Here's how the part is built. I have some questions about the finished solid (model axes, mm). A direction names the side the tool comes from. Coordinates: 2 decimals unless noted, no trailing zeros. Write each loop counter-clockwise with the first axis right and the second up, starting at its lowest first coordinate (ties: lowest second). Pieces come first, ordered by that corner, then holes. Notation, with made-up numbers: M -18,-26 L 26,-26 A30 cw 26,11 Z; hole C -29.75,-35.75 d7. An arc over 180 degrees is marked long. Use one line per item in the form item = value. Start each with the question number.
1. I want a section at A-A, the plane z = 0. List the corners of the cut face in (x, y) for me.
2. I want a section at B-B, the plane y = 3.1. List the corners of the cut face in (x, z) for me, plus the area to 3 significant figures.
3. On a 3-axis mill with a long thin cutter (end or side, diameter ignored), from which of +Z, -Z, +X, -X, +Y, -Y can I reach the whole of each face in a straight line? I mean faces 4 (the face through (-164.45, 1.29, -2.54)), 5 (the face through (-61.05, 2.48, -0.25)). Say none if no direction works.
4. Thinking about a two-plate mould opening in Z: for faces 1 (the face through (-170.5, 2.105, 0.1)), 2 (the face through (-115, 0.505, 0)), 3 (the face through (-116, 2, -6)), which applies, released by +Z, released by -Z, zero draft, split by the parting line, or undercut?
5. I'm going to push flat-ended pins straight in: pin 1 Ø4.5 at (x, z) = (-62.95, 0) entering from -Y; pin 2 Ø2.5 at (x, z) = (-168.43, 0) entering from -Y; pin 3 Ø5.5 at (x, z) = (-168.43, 0) entering from -Y. Where does each tip first touch, or does it pass through?
6. Please list where these lines run through material, in increasing order: line 1 along X through (y, z) = (1.65, 0); line 2 along X through (y, z) = (2.8, 0.25); line 3 along Z through (x, y) = (-169, 4.15). Write a range as [from, to].
from build123d import *

# Parameters (mm, degrees)
SKETCH1_R           = 2.4
BOSS_EXTRUDE1_DEPTH = 5
SKETCH2_R           = 5.9
CUT_EXTRUDE1_DEPTH  = 2
SCALE1_SCALE        = 0.8


with BuildPart() as part:
    # Sketch1 → Boss-Extrude1 (new body)
    with BuildSketch(Plane(origin=(0, 0, 0), x_dir=(1, 0, 0), z_dir=(0, 1, 0))):
        with BuildLine():
            Line((-181.84579044, 7.5), (-50, 7.5))
            ThreePointArc((-50, 7.5), (-42.5, 0), (-50, -7.5))
            Line((-50, -7.5), (-181.84579044, -7.5))
            ThreePointArc((-181.84579044, -7.5), (-189.34579044, 0), (-181.84579044, 7.5))
        make_face()
        with Locations(Location((-181.84579044, 0, 0), (0, 0, 270))):
            Circle(SKETCH1_R, mode=Mode.SUBTRACT)
        with Locations(Location((-50, 0, 0), (0, 0, 270))):
            Circle(SKETCH1_R, mode=Mode.SUBTRACT)
    extrude(amount=BOSS_EXTRUDE1_DEPTH)

    # Sketch2 → Cut-Extrude1 (cut)
    with BuildSketch(Plane.XZ):
        with Locations(Location((-181.84579044, 0, 0), (0, 0, 270))):
            Circle(SKETCH2_R)
    extrude(amount=-CUT_EXTRUDE1_DEPTH, mode=Mode.SUBTRACT)


with BuildPart() as part_1:
    # Scale1: scaled about (-114.766854611, 2.52630438, 0)
    add(part.part.scale(SCALE1_SCALE).moved(Location((-22.953370922, 0.505260876, 0))))


solid = part_1.part
Answer list:
q1.outline = M -174.43,0.51 L -173.15,0.51 L -173.15,2.11 L -170.35,2.11 L -170.35,4.51 L -174.43,4.51 Z; M -166.51,2.11 L -163.71,2.11 L -163.71,0.51 L -64.87,0.51 L -64.87,4.51 L -166.51,4.51 Z; M -61.03,0.51 L -56.95,0.51 L -56.95,4.51 L -61.03,4.51 Z
q2.outline = M -168.43,-6 L -62.95,-6 A6 ccw -62.95,6 L -168.43,6 A6 ccw Z; hole C -168.43,0 d3.84; hole C -62.95,0 d3.84
q2.area = 1,360 mm²
q3.face_4 = -Y
q3.face_5 = +Y, -Y
q4.face_1 = undercut
q4.face_2 = zero draft
q4.face_3 = released by -Z
q5.pin_1 = 0.51
q5.pin_2 = through
q5.pin_3 = 2.11
q6.line_1 = [-174.43, -173.15], [-163.71, -64.87], [-61.03, -56.95]
q6.line_2 = [-174.42, -170.33], [-166.53, -64.86], [-61.05, -56.96]
q6.line_3 = [-5.97, -1.83], [1.83, 5.97]
